from build123d import *

# Parameters (mm, degrees)
SKETCH1_W                                = 200
SKETCH1_H                                = 100
BOSS_EXTRUDE1_DEPTH                      = 15
FILLET1_R                                = 10
CBORE_FOR_M10_HEX_HEAD_BOLT1_D           = 11
CBORE_FOR_M10_HEX_HEAD_BOLT1_CBORE_D     = 21.475
CBORE_FOR_M10_HEX_HEAD_BOLT1_CBORE_DEPTH = 6.4
F_8_0MM_DOWEL_HOLE1_D                    = 8
CHAMFER1_SIZE                            = 1


with BuildPart() as part:
    # Sketch1 → Boss-Extrude1 (new body)
    with BuildSketch(Plane.XY):
        Rectangle(SKETCH1_W, SKETCH1_H)
    extrude(amount=BOSS_EXTRUDE1_DEPTH)

    # Fillet1
    fillet1_edges = [part.edges().sort_by_distance(p)[0] for p in [
        (100, -50, 7.5),
        (-100, -50, 7.5),
        (-100, 50, 7.5),
        (100, 50, 7.5),
    ]]
    fillet(fillet1_edges, radius=FILLET1_R)

    # CBORE for M10 Hex Head Bolt1 (through all)
    with Locations(Plane.XY.offset(15)):
        with Locations((48.132684833, 22.427148815), (48.132684833, -19.595814413)):
            CounterBoreHole(CBORE_FOR_M10_HEX_HEAD_BOLT1_D / 2, CBORE_FOR_M10_HEX_HEAD_BOLT1_CBORE_D / 2, CBORE_FOR_M10_HEX_HEAD_BOLT1_CBORE_DEPTH)

    # Ø8.0mm Dowel Hole1 (through all)
    with Locations(Plane.XY.offset(15)):
        with Locations((48.281702433, 0)):
            Hole(F_8_0MM_DOWEL_HOLE1_D / 2)

    # Chamfer1
    chamfer1_edges = [part.edges().sort_by_distance(p)[0] for p in [
        (0, 50, 0),
        (0, 50, 15),
        (100, 0, 0),
        (0, -50, 0),
        (-100, 0, 0),
        (-97.071067812, -47.071067812, 0),
        (-97.071067812, 47.071067812, 0),
        (97.071067812, -47.071067812, 0),
        (97.071067812, 47.071067812, 0),
        (100, 0, 15),
        (-100, 0, 15),
        (0, -50, 15),
        (-97.071067812, -47.071067812, 15),
        (-97.071067812, 47.071067812, 15),
        (97.071067812, -47.071067812, 15),
        (97.071067812, 47.071067812, 15),
    ]]
    chamfer(chamfer1_edges, length=CHAMFER1_SIZE)


solid = part.part
Can you work these out from the model? Positions are in its coordinate system, mm. A direction names the side the tool comes from. Round coordinates to 2 decimals unless told otherwise and drop trailing zeros. Write each loop counter-clockwise with the first axis right and the second up, starting at its lowest first coordinate (ties: lowest second). Pieces come first, ordered by that corner, then holes. Notation, with made-up numbers: (50.25, -32) -> (69.25, -32) arc R16 cw to (69.25, -3) -> close; hole circle Ø6 at (55.25, -31). An arc over 180 degrees is marked (long way). Use one line per item in the form item = value. Start each with the question number.
Q1. I'm going to push a flat-ended pin straight in: P1, Ø23.5, axis at x = 43.5, y = 22.5, coming from the +Z side. Where does the tip first touch, or does it pass through?
Q2. Imagine slicing it at B-B (z = 6.75). Please give me the cut outline in (x, y), then the cut area to 3 significant figures.
Q3. Imagine slicing it at A-A (y = 0). Please give me the cut outline in (x, z), then the cut area to 3 significant figures.
Q4. Which directions (+Z, -Z, +X, -X, +Y, -Y) give clear straight access to the entire face, cutting with the end or side of a thin tool? Please do faces 4 (the face through (43, 25, 8.6)), 5 (the face through (-96.558, 46.415, 0.174)).
Q5. We'd pull the mould along X, two halves only. Please class faces 1 (the face through (-97.15, -46.99, 7.59)), 2 (the face through (53.627, -19.354, 4.24)), 3 (the face through (96.415, 46.558, 0.174)): +X half, -X half, draft (parallel to the pull), parting line (faces both ways), or undercut.
Q6. Imagine slicing it at C-C (y = 31). Please give me the cut outline in (x, z), then the cut area to 3 significant figures.
Q7. If I drill on probe 1 along X at (y, z) = (-22, 5.75); probe 2 along X at (y, z) = (-3, 8.25); probe 3 along Z at (x, y) = (48.5, -14), over which ranges is the centre line in solid material (lowest first)? Write a range as [from, to].
Worked out:
q1.P1 = 15
q2.outline = (-100, -40) arc R10 ccw to (-90, -50) -> (90, -50) arc R10 ccw to (100, -40) -> (100, 40) arc R10 ccw to (90, 50) -> (-90, 50) arc R10 ccw to (-100, 40) -> close; hole circle Ø11 at (48.13, -19.6); hole circle Ø11 at (48.13, 22.43); hole circle Ø8 at (48.28, 0)
q2.area = 19,700 mm^2
q3.outline = (-100, 1) -> (-99, 0) -> (44.28, 0) -> (44.28, 15) -> (-99, 15) -> (-100, 14) -> close; (52.28, 0) -> (99, 0) -> (100, 1) -> (100, 14) -> (99, 15) -> (52.28, 15) -> close
q3.area = 2,880 mm^2
q4.face_4 = +Z
q4.face_5 = -Z, -X, +Y
q5.face_1 = -X half
q5.face_2 = undercut
q5.face_3 = +X half
q6.outline = (-100, 1) -> (-99, 0) -> (99, 0) -> (100, 1) -> (100, 14) -> (99, 15) -> (54.6, 15) -> (54.6, 8.6) -> (41.67, 8.6) -> (41.67, 15) -> (-99, 15) -> (-100, 14) -> close
q6.area = 2,920 mm^2
q7.probe_1 = [-100, 43.19], [53.08, 100]
q7.probe_2 = [-100, 45.64], [50.93, 100]
q7.probe_3 = [0, 8.6]
